Input: part model. Units: mm. Frame: model coordinates. A direction names the side the tool comes from. Give positions to 0.01 mm unless a question says otherwise; leave off trailing zeros. Loops run counter-clockwise (first coordinate to the right, second up) from the corner with the lowest first, then second, coordinate; pieces in that order, holes last. Notation, with made-up numbers: (57.5, 74) - (98.5, 74) arc R25 ccw to (98.5, 103) - close; hole circle Ø4 at (2.5, 35). An arc over 180 degrees is marked (long way). Answer as a JSON object with one key per item and string values.
from build123d import *

# Parameters (mm, degrees)
BOSS_EXTRUDE2_DEPTH     = 30
CUT_EXTRUDE1_DEPTH      = 173.336879396
CUT_EXTRUDE1_DEPTH_BACK = 15
SKETCH4_W               = 10
SKETCH4_H               = 5
BOSS_EXTRUDE3_DEPTH     = 10
CHAMFER1_SIZE           = 2
SKETCH6_W               = 5
SKETCH6_H               = 10
CUT_EXTRUDE2_DEPTH      = 10
FILLET1_R               = 1


with BuildPart() as part:
    # Sketch1 → Boss-Extrude2 (new body)
    with BuildSketch(Plane.XY):
        with BuildLine():
            Line((0, 100), (0, 120))
            ThreePointArc((0, 120), (-103.923048454, 60), (-103.923048454, -60))
            Line((-103.923048454, -60), (-86.602540378, -50))
            ThreePointArc((-86.602540378, -50), (-86.602540378, 50), (0, 100))
        make_face()
    extrude(amount=BOSS_EXTRUDE2_DEPTH)

    # Sketch3 → Cut-Extrude1 (cut, two sides: drawn at the far end of the back side and taken through both)
    with BuildSketch(Plane.XY.offset(30).offset(-CUT_EXTRUDE1_DEPTH_BACK)):
        with BuildLine():
            ThreePointArc((-90.932667397, -52.5), (-90.932667397, 52.5), (0, 105))
            Line((0, 105), (0, 115))
            ThreePointArc((0, 115), (-99.592921435, 57.5), (-99.592921435, -57.5))
            Line((-99.592921435, -57.5), (-90.932667397, -52.5))
        make_face()
    extrude(amount=CUT_EXTRUDE1_DEPTH + CUT_EXTRUDE1_DEPTH_BACK, mode=Mode.SUBTRACT)

    # Sketch4 → Boss-Extrude3 (add)
    with BuildSketch(Plane(origin=(0, 0, 0), x_dir=(0, 0, -1), z_dir=(1, 0, 0))):
        with Locations((-7.5, 109.798266437)):
            Rectangle(SKETCH4_W, SKETCH4_H)
    extrude(amount=BOSS_EXTRUDE3_DEPTH)

    # Chamfer1
    chamfer1_edges = [part.edges().sort_by_distance(p)[0] for p in [
        (10, 109.798266437, 2.5),
        (10, 112.298266437, 7.5),
        (10, 109.798266437, 12.5),
        (10, 107.298266437, 7.5),
    ]]
    chamfer(chamfer1_edges, length=CHAMFER1_SIZE)

    # Sketch6 → Cut-Extrude2 (cut)
    with BuildSketch(Plane(origin=(0, 0, 0), x_dir=(0.8660254037844363, 0.5000000000000042, 0), z_dir=(0.5000000000000041, -0.8660254037844362, 0))):
        with Locations((-109.951600937, 7.5)):
            Rectangle(SKETCH6_W, SKETCH6_H)
    extrude(amount=-CUT_EXTRUDE2_DEPTH, mode=Mode.SUBTRACT)

    # Fillet1
    fillet1_edges = [part.edges().sort_by_distance(p)[0] for p in [
        (-86.602540378, 50, 30),
        (-103.923048454, 60, 30),
    ]]
    fillet(fillet1_edges, radius=FILLET1_R)


solid = part.part
Item 1: Cut plane A-A (z = 27). Return loops of the section in (x, y), then the cut area to 3 significant figures.
Geometry check:
{"outline": "(-103.92, -60) - (-99.59, -57.5) arc R115 cw to (0, 115) - (0, 120) arc R120 ccw to start; (-90.93, -52.5) - (-86.6, -50) arc R100 cw to (0, 100) - (0, 105) arc R105 ccw to start", "area": "2,300 mm2"}
Item 2: Access query for faces 4 (the face through (4, 110, 12.5)), 5 (the face through (-100.251, -46.333, 7.57)), 6 (the face through (4, 107.298, 8)), 7 (the face through (4, 112.298, 8)). Directions: +Z, -Z, +X, -X, +Y, -Y. A direction counts if a zero-diameter tool reaches every point of the face in a straight line with its end or side. Return the directions, or none.
Geometry check:
{"face 4": "+Z, +X, +Y, -Y", "face 5": "none", "face 6": "+Z, -Z, +X, -Y", "face 7": "+Z, -Z, +X, +Y"}
Item 3: Contact query for flat-ended pins moving along their axis: P1, Ø4.5, axis at x = -97.5, y = -53.5, coming from the +Z side; P2, Ø4, axis at x = 3, z = 9.5, coming from the +Y side; P3, Ø5, axis at x = -57.5, z = 17, coming from the -Y side. Output: stop coordinate, or through.
Geometry check:
{"P1": "stops at z = 15", "P2": "stops at y = 112.3", "P3": "stops at y = 80"}
Item 4: Mould query, pull axis Z, two halves, no side actions, for faces 1 (the face through (-103.03, 61.52, 14.3)), 2 (the face through (-98, -51, 12.5)), 3 (the face through (-91, 44, 0)). Classes: released by +Z, released by -Z, zero draft, split by the parting line, or undercut.
Geometry check:
{"face 1": "zero draft", "face 2": "undercut", "face 3": "released by -Z"}
Item 5: Cut plane C-C (x = 2). Return loops of the section in (y, z), then the cut area to 3 significant figures.
Geometry check:
{"outline": "(107.3, 2.5) - (112.3, 2.5) - (112.3, 12.5) - (107.3, 12.5) - close", "area": "50.0 mm2"}
Item 6: Material intervals for line 1 (Y direction, x = -91, z = 17); line 2 (X direction, y = -42, z = 18); line 3 (Y direction, x = -18, z = 26.5), sorted ascending. Write a range as [from, to].
Geometry check:
{"line 1": "y = [-52.38, -41.46], [41.46, 52.38], [70.31, 78.22]", "line 2": "x = [-112.41, -107.06], [-96.23, -90.75]", "line 3": "y = [98.37, 103.45], [113.58, 118.64]"}
Item 7: Cut plane B-B (z = 8.5). Return loops of the section in (x, y), then the cut area to 3 significant figures.
Geometry check:
{"outline": "(-103.92, -60) - (-97.39, -56.23) - (-102.39, -47.57) - (-98.06, -45.07) - (-93.06, -53.73) - (-86.6, -50) arc R100 cw to (0, 100) - (0, 107.3) - (8, 107.3) - (10, 109.3) - (10, 110.3) - (8, 112.3) - (0, 112.3) - (0, 120) arc R120 ccw to start", "area": "4,600 mm2"}
